Part model, mm, in its own coordinate system. Give positions to 0.01 mm unless a question says otherwise; leave off trailing zeros. Order: outer loops, then holes, each group sorted by start corner. A loop starts at its lowest first (then second) coordinate and runs counter-clockwise, first axis right, second up. Notation, with made-up numbers: M 26,-38 L 71,-38 A9 cw 71,-24 Z; hole C 63.5,9.5 d6. An arc over 180 degrees is marked long. Answer as a JSON object with one key per item and string values.
from build123d import *

# Parameters (mm, degrees)
SKETCH1_R                      = 100
BOSS_EXTRUDE1_DEPTH            = 7.5
CBORE_FOR_M3_SHCS1_D           = 3.4
CBORE_FOR_M3_SHCS1_DEPTH       = 7.5
CBORE_FOR_M3_SHCS1_CBORE_D     = 6.5
CBORE_FOR_M3_SHCS1_CBORE_DEPTH = 3
CBORE_FOR_M3_SHCS1_TIP         = 1.021463052
CBORE_FOR_M3_SHCS2_D           = 3.6
CBORE_FOR_M3_SHCS2_DEPTH       = 7.5
CBORE_FOR_M3_SHCS2_CBORE_D     = 6.5
CBORE_FOR_M3_SHCS2_CBORE_DEPTH = 3
CBORE_FOR_M3_SHCS2_TIP         = 1.081549114


with BuildPart() as part:
    # Sketch1 → Boss-Extrude1 (new body)
    with BuildSketch(Plane(origin=(0, 0, 0), x_dir=(1, 0, 0), z_dir=(0, 1, 0))):
        with Locations(Location((0, 0, 0), (0, 0, 270))):
            Circle(SKETCH1_R)
    extrude(amount=BOSS_EXTRUDE1_DEPTH)

    # CBORE for M3 SHCS1
    with Locations(Plane(origin=(0, 0, 0), x_dir=(-1, 0, 0), z_dir=(0, -1, 0))):
        with Locations((0, -92.5), (-65.40737726, -65.40737726), (-92.5, 0), (-65.40737726, 65.40737726), (0, 92.5), (65.40737726, 65.40737726), (92.5, 0), (65.40737726, -65.40737726)):
            CounterBoreHole(CBORE_FOR_M3_SHCS1_D / 2, CBORE_FOR_M3_SHCS1_CBORE_D / 2, CBORE_FOR_M3_SHCS1_CBORE_DEPTH, depth=CBORE_FOR_M3_SHCS1_DEPTH)
            with Locations((0, 0, -(CBORE_FOR_M3_SHCS1_DEPTH + CBORE_FOR_M3_SHCS1_TIP / 2))):  # 118° drill point
                Cone(0, CBORE_FOR_M3_SHCS1_D / 2, CBORE_FOR_M3_SHCS1_TIP, mode=Mode.SUBTRACT)

    # CBORE for M3 SHCS2
    with Locations(Plane(origin=(0, 0, 0), x_dir=(-1, 0, 0), z_dir=(0, -1, 0))):
        with Locations((-53, 34), (53, 34), (53, -34), (-53, -34)):
            CounterBoreHole(CBORE_FOR_M3_SHCS2_D / 2, CBORE_FOR_M3_SHCS2_CBORE_D / 2, CBORE_FOR_M3_SHCS2_CBORE_DEPTH, depth=CBORE_FOR_M3_SHCS2_DEPTH)
            with Locations((0, 0, -(CBORE_FOR_M3_SHCS2_DEPTH + CBORE_FOR_M3_SHCS2_TIP / 2))):  # 118° drill point
                Cone(0, CBORE_FOR_M3_SHCS2_D / 2, CBORE_FOR_M3_SHCS2_TIP, mode=Mode.SUBTRACT)


solid = part.part
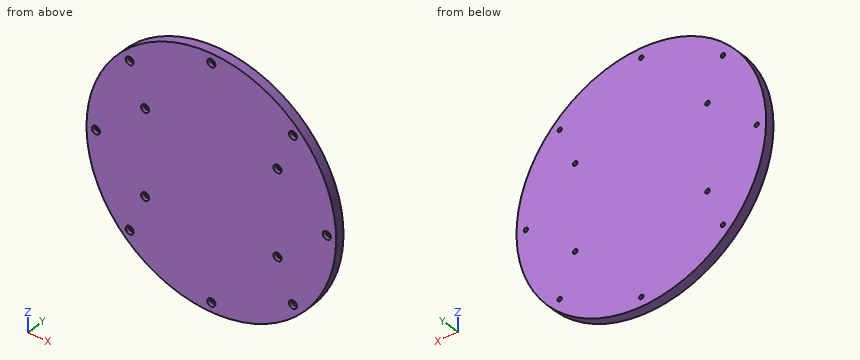
1. Cut at B-B on z = -76.5. Give the cut face in (x, y).
Worked answers:
{"outline": "M -64.4,0 L 64.4,0 L 64.4,7.5 L -64.4,7.5 Z"}
2. Cut at A-A on z = 76. Give the cut face in (x, y), plus the area to 3 significant figures.
Worked answers:
{"outline": "M -64.99,0 L 64.99,0 L 64.99,7.5 L -64.99,7.5 Z", "area": "975 mm^2"}
3. Probe line 1 along Z through (x, y) = (67, 2.5); line 2 along X through (y, z) = (2.75, -37). List the from-to ranges inside material, lowest first.
Worked answers:
{"line 1": "z = -74.24 to -68.24, -62.57 to 62.57, 68.24 to 74.24", "line 2": "x = -92.9 to -54.25, -51.75 to 51.75, 54.25 to 92.9"}
4. Pin check, flat tips, straight feed: P1, Ø3, axis at x = -53, z = 34, coming from the -Y side; P2, Ø4, axis at x = 28.5, y = 4, coming from the -Z side; P3, Ø2, axis at x = 51.5, z = 32.5, coming from the -Y side; P4, Ø3, axis at y = 5, z = -26.5, coming from the +X side. Stop position of each tip, or through.
Worked answers:
{"P1": "passes through", "P2": "stops at z = -96.42", "P3": "stops at y = 3", "P4": "stops at x = 96.82"}
